Read the model definition and answer for the solid it produces. Units are mm, in the model's axes. Face numbers are marked on the shaded views. A direction names the side the tool comes from. Round coordinates to 2 decimals unless told otherwise and drop trailing zeros. Loops run counter-clockwise (first coordinate to the right, second up) from the corner with the lowest first, then second, coordinate; pieces in that order, holes last. Notation, with made-up numbers: (2.5, 59) - (24.5, 59) arc R5 ccw to (24.5, 63) - close; hole circle Ø9 at (-14, 22.25). An arc over 180 degrees is marked (long way). Answer as CSV lines item,"result".
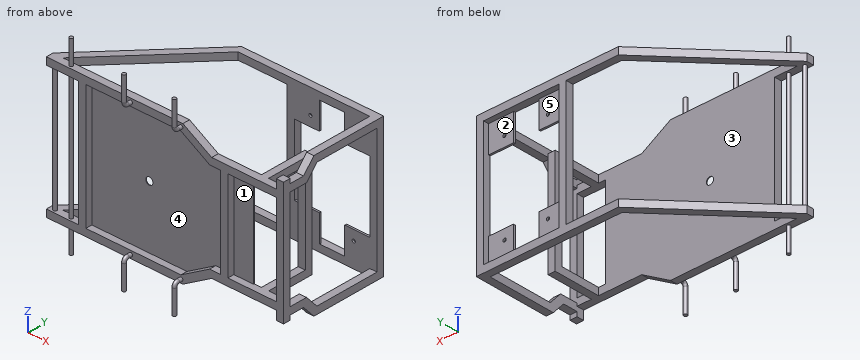
```python
from build123d import *

# Parameters (mm, degrees)
BOSS_EXTRUDE1_DEPTH = 10
SKETCH2_R           = 5
SKETCH2_W           = 20
SKETCH2_H           = 20
BOSS_EXTRUDE2_DEPTH = 175
SKETCH3_R           = 5
BOSS_EXTRUDE3_DEPTH = 260
SKETCH4_R           = 5
SKETCH5_W           = 30
SKETCH5_H           = 20
CUT_EXTRUDE1_DEPTH  = 20
SKETCH6_W           = 55
SKETCH6_H           = 250
BOSS_EXTRUDE4_DEPTH = 2
SKETCH7_R           = 10
CUT_EXTRUDE2_DEPTH  = 30
SKETCH8_W           = 20
SKETCH8_H           = 150
BOSS_EXTRUDE5_DEPTH = 145
SKETCH9_W           = 250
SKETCH9_H           = 130
CUT_EXTRUDE3_DEPTH  = 20
SKETCH10_W          = 25
SKETCH10_H          = 20
BOSS_EXTRUDE6_DEPTH = 20
BOSS_EXTRUDE7_DEPTH = 20
SKETCH14_W          = 20
SKETCH14_H          = 20
BOSS_EXTRUDE8_DEPTH = 175
SKETCH15_R          = 4.5
BOSS_EXTRUDE9_DEPTH = 5


with BuildPart() as part:
    # Sketch1 → Boss-Extrude1 (new, symmetric)
    with BuildSketch(Plane(origin=(0, 0, 0), x_dir=(1, 0, 0), z_dir=(0, 1, 0))):
        Polygon((-330, 192.5), (50, 192.5), (130, 145), (330, 145), (330, 125), (330, -125), (330, -145), (130, -145), (50, -192.5), (-330, -192.5), (-330, -172.5), (44.50990723, -172.5), (124.50990723, -125), (310, -125), (310, 125), (124.50990723, 125), (44.50990723, 172.5), (-330, 172.5), align=None)
    extrude(amount=BOSS_EXTRUDE1_DEPTH, both=True)

    # Sketch2 → Boss-Extrude2 (add, symmetric)
    with BuildSketch(Plane.XY):
        with Locations(Location((-315, 0, 0), (0, 0, 180))):
            Circle(SKETCH2_R)
        with Locations((-230, 0)):
            Rectangle(SKETCH2_W, SKETCH2_H)
        with Locations((165, 0)):
            Rectangle(SKETCH2_W, SKETCH2_H)
    extrude(amount=BOSS_EXTRUDE2_DEPTH, both=True)

    # Sketch3 → Boss-Extrude3 (add, symmetric)
    with BuildSketch(Plane.XY):
        with Locations((-270, 0)):
            Circle(SKETCH3_R)
    extrude(amount=BOSS_EXTRUDE3_DEPTH, both=True)

    # Sweep1: sweep along a curve in space
    with BuildLine() as sweep1_path:
        Line((-95, -10, 182.5), (-95, -20, 182.5))
        ThreePointArc((-95, -20, 182.5), (-95, -27.071067812, 185.428932188), (-95, -30, 192.5))
        Line((-95, -30, 192.5), (-95, -30, 260))
    # Sketch4 → Sweep1 (sweep)
    with BuildSketch(Plane.XZ.offset(10)):
        with Locations((-95, 182.5)):
            Circle(SKETCH4_R)
        with Locations((45, 182.5)):
            Circle(SKETCH4_R)
    sweep1 = sweep(path=sweep1_path.line)

    # Mirror1: Sweep1 across plane
    add(sweep1.mirror(Plane.XY))

    # Sketch5 → Cut-Extrude1 (cut)
    with BuildSketch(Plane(origin=(175, 0, 0), x_dir=(0, 0, -1), z_dir=(1, 0, 0))):
        with Locations((-160, 0)):
            Rectangle(SKETCH5_W, SKETCH5_H)
        with Locations((160, 0)):
            Rectangle(SKETCH5_W, SKETCH5_H)
    extrude(amount=-CUT_EXTRUDE1_DEPTH, mode=Mode.SUBTRACT)

    # Sketch6 → Boss-Extrude4 (add)
    with BuildSketch(Plane(origin=(0, 10, 0), x_dir=(1, 0, 0), z_dir=(0, 1, 0))):
        Polygon((-220, -172.5), (-220, 172.5), (44.50990723, 172.5), (124.50990723, 125), (155, 125), (155, -125), (124.50990723, -125), (44.50990723, -172.5), align=None)
        with Locations((202.5, 0)):
            Rectangle(SKETCH6_W, SKETCH6_H)
    extrude(amount=-BOSS_EXTRUDE4_DEPTH)

    # Sketch7 → Cut-Extrude2 (cut)
    with BuildSketch(Plane(origin=(0, 10, 0), x_dir=(1, 0, 0), z_dir=(0, 1, 0))):
        with Locations(Location((-60, 0, 0), (0, 0, 270))):
            Circle(SKETCH7_R)
    extrude(amount=-CUT_EXTRUDE2_DEPTH, mode=Mode.SUBTRACT)

    # Sketch8 → Boss-Extrude5 (add, symmetric)
    with BuildSketch(Plane.XY):
        with Locations((260, 65)):
            Rectangle(SKETCH8_W, SKETCH8_H)
    extrude(amount=BOSS_EXTRUDE5_DEPTH, both=True)

    # Sketch9 → Cut-Extrude3 (cut)
    with BuildSketch(Plane(origin=(270, 0, 0), x_dir=(0, 0, -1), z_dir=(1, 0, 0))):
        with Locations((0, 55)):
            Rectangle(SKETCH9_W, SKETCH9_H)
    extrude(amount=-CUT_EXTRUDE3_DEPTH, mode=Mode.SUBTRACT)

    # Sketch10 → Boss-Extrude6 (add)
    with BuildSketch(Plane(origin=(330, 0, 0), x_dir=(0, 0, -1), z_dir=(1, 0, 0))):
        Polygon((-157.5, 10), (-157.5, 50), (-192.5, 80.996688705), (-192.5, 290), (192.5, 290), (192.5, 80.996688705), (157.5, 50), (157.5, 10), (137.5, 10), (137.5, 59.003311295), (172.5, 90), (172.5, 270), (-172.5, 270), (-172.5, 90), (-137.5, 59.003311295), (-137.5, 10), align=None)
        with Locations((157.5, 0)):
            Rectangle(SKETCH10_W, SKETCH10_H)
        with Locations((-157.5, 0)):
            Rectangle(SKETCH10_W, SKETCH10_H)
    extrude(amount=-BOSS_EXTRUDE6_DEPTH)

    # Sketch13 → Boss-Extrude7 (add)
    with BuildSketch(Plane(origin=(0, 0, -192.5), x_dir=(-1, 0, 0), z_dir=(0, 0, -1))):
        Polygon((-310, 290), (65, 290), (330, 10), (302.462919248, 10), (56.391490677, 270), (-310, 270), align=None)
    boss_extrude7 = extrude(amount=-BOSS_EXTRUDE7_DEPTH)

    # Mirror2: Boss-Extrude7 across plane
    add(boss_extrude7.mirror(Plane.XY))

    # Sketch14 → Boss-Extrude8 (add, symmetric)
    with BuildSketch(Plane.XY):
        with Locations((90, 280)):
            Rectangle(SKETCH14_W, SKETCH14_H)
    extrude(amount=BOSS_EXTRUDE8_DEPTH, both=True)

    # Sketch15 → Boss-Extrude9 (add)
    # profile 1 of 4: a face of its own
    with BuildSketch(Plane(origin=(0, 270, 0), x_dir=(-1, 0, 0), z_dir=(0, -1, 0))):
        with BuildLine():
            Line((-310, 97.5), (-241, 97.5))
            ThreePointArc((-241, 97.5), (-240.292893219, 97.792893219), (-240, 98.5))
            Line((-240, 98.5), (-240, 172.5))
            Line((-240, 172.5), (-310, 172.5))
            Line((-310, 172.5), (-310, 97.5))
        make_face()
        with Locations(Location((-265.332009498, 125.279552898, 0), (0, 0, 270))):
            Circle(SKETCH15_R, mode=Mode.SUBTRACT)
    # profile 2 of 4: a face of its own
    with BuildSketch(Plane(origin=(0, 270, 0), x_dir=(-1, 0, 0), z_dir=(0, -1, 0))):
        with BuildLine():
            Line((-100, 172.5), (-170, 172.5))
            Line((-170, 172.5), (-170, 98.5))
            ThreePointArc((-170, 98.5), (-169.707106781, 97.792893219), (-169, 97.5))
            Line((-169, 97.5), (-100, 97.5))
            Line((-100, 97.5), (-100, 172.5))
        make_face()
        with Locations(Location((-144.667990502, 125.279552898, 0), (0, 0, 90))):
            Circle(SKETCH15_R, mode=Mode.SUBTRACT)
    # profile 3 of 4: a face of its own
    with BuildSketch(Plane(origin=(0, 270, 0), x_dir=(-1, 0, 0), z_dir=(0, -1, 0))):
        with BuildLine():
            Line((-310, -172.5), (-310, -97.5))
            Line((-310, -97.5), (-241, -97.5))
            ThreePointArc((-241, -97.5), (-240.292893219, -97.792893219), (-240, -98.5))
            Line((-240, -98.5), (-240, -172.5))
            Line((-240, -172.5), (-310, -172.5))
        make_face()
        with Locations(Location((-265.332009498, -125.279552898, 0), (0, 0, 90))):
            Circle(SKETCH15_R, mode=Mode.SUBTRACT)
    # profile 4 of 4: a face of its own
    with BuildSketch(Plane(origin=(0, 270, 0), x_dir=(-1, 0, 0), z_dir=(0, -1, 0))):
        with BuildLine():
            Line((-100, -97.5), (-169, -97.5))
            ThreePointArc((-169, -97.5), (-169.707106781, -97.792893219), (-170, -98.5))
            Line((-170, -98.5), (-170, -172.5))
            Line((-170, -172.5), (-100, -172.5))
            Line((-100, -172.5), (-100, -97.5))
        make_face()
        with Locations(Location((-144.667990502, -125.279552898, 0), (0, 0, 270))):
            Circle(SKETCH15_R, mode=Mode.SUBTRACT)
    extrude(amount=-BOSS_EXTRUDE9_DEPTH)


solid = part.part
```
1) Each of these flat-tipped pins is pushed along its axis until it touches: P1, Ø6, axis at x = -67, z = 56, coming from the +Y side; P2, Ø16, axis at y = 277.5, z = 1.5, coming from the -X side; P3, Ø8, axis at x = 79, z = 16, coming from the -Y side; P4, Ø12, axis at y = 195, z = -202.5, coming from the +X side. Where does it stop, or does it pass through?
Entries:
P1,"stops at y = 10"
P2,"stops at x = 80"
P3,"stops at y = 8"
P4,"passes through"
2) A cutting plane is placed at D-D, the plane z = -225. Determine the outline of the cut face in (x, y).
Entries:
outline,"circle Ø10 at (-270, 0); circle Ø10 at (-95, -30); circle Ø10 at (45, -30)"
3) A cutting plane is placed at C-C, the plane y = 189. Determine the outline of the cut face in (x, z).
Entries:
outline,"(-160.59, -192.5) - (-133.05, -192.5) - (-133.05, -172.5) - (-160.59, -172.5) - close; (-160.59, 172.5) - (-133.05, 172.5) - (-133.05, 192.5) - (-160.59, 192.5) - close; (310, -192.5) - (330, -192.5) - (330, -172.5) - (310, -172.5) - close; (310, 172.5) - (330, 172.5) - (330, 192.5) - (310, 192.5) - close"
4) A cutting plane is placed at B-B, the plane x = -188. Determine the outline of the cut face in (y, z), plus the area to 3 significant figures.
Entries:
outline,"(-10, -192.5) - (10, -192.5) - (10, 192.5) - (-10, 192.5) - (-10, 172.5) - (8, 172.5) - (8, -172.5) - (-10, -172.5) - close; (130.94, -192.5) - (160.04, -192.5) - (160.04, -172.5) - (130.94, -172.5) - close; (130.94, 172.5) - (160.04, 172.5) - (160.04, 192.5) - (130.94, 192.5) - close"
area,"2,650 mm^2"
5) A tool of negligible diameter and unlimited length cuts with its end or side. For the marked faces 1 and 2, from which of +Z, -Z, +X, -X, +Y, -Y can it reach the whole face along a straight path? Write none if from no direction.
Entries:
face 1,"-Y"
face 2,"+Y"
6) The mould has two halves that part along Y. Classify the marked faces 3, 4 and 5: pulls with the +Y half, pulls with the -Y half, needs draft (parallel to the pull), parting line crosses it, or undercut.
Entries:
face 3,"undercut"
face 4,"pulls with the -Y half"
face 5,"pulls with the +Y half"
7) A cutting plane is placed at A-A, the plane z = -112.5. Count the separate pieces of the cut face and the enclosed holes in it, plus the area to 3 significant figures.
Entries:
separate pieces,"7"
enclosed holes,"0"
area,"4,120 mm^2"
8) Find the intervals of material crossed by line 1 (Z direction, x = -125.5, y = 2.5); line 2 (Y direction, x = -180, z = 39.5); line 3 (Y direction, x = 29, z = 176), in increasing order.
Entries:
line 1,"z = -192.5 to -172.5, 172.5 to 192.5"
line 2,"y = 8 to 10"
line 3,"y = -10 to 10, 270 to 290"
